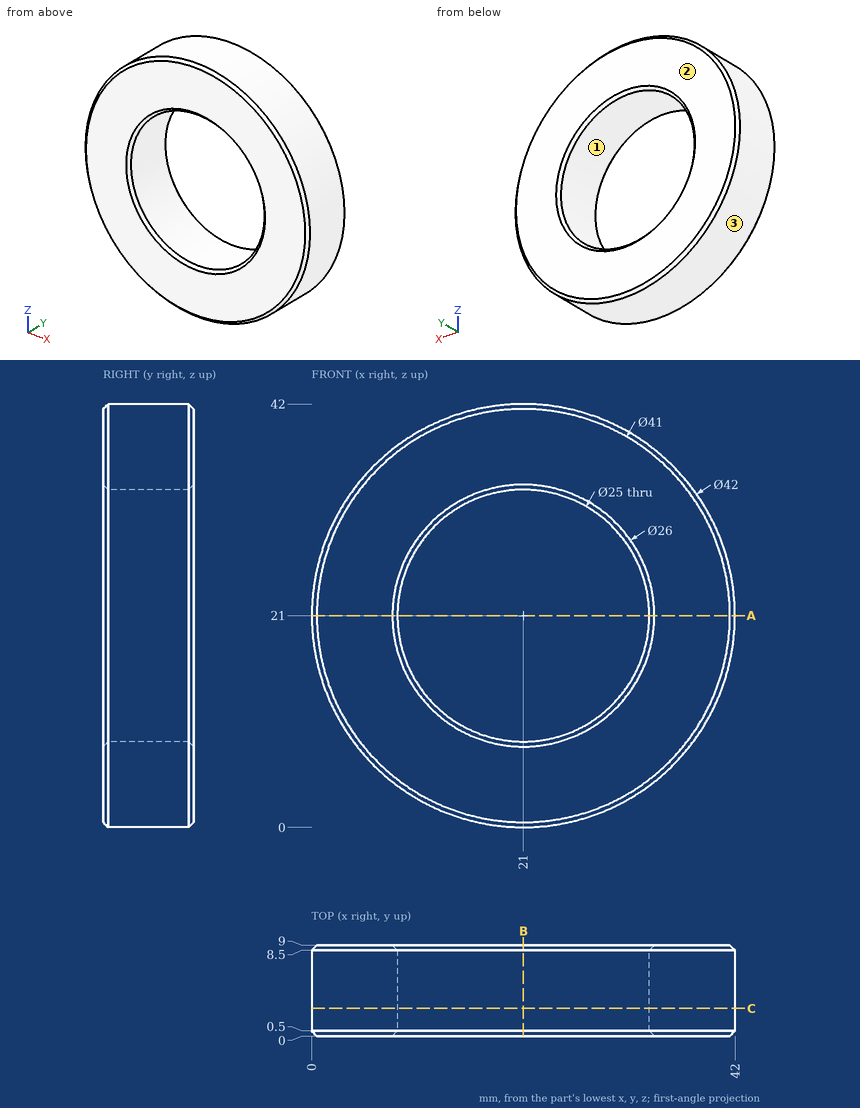
Study the drawing (mm; zero at the part's minimum x, y, z) and answer. Coordinates: 2 decimals unless noted, no trailing zeros. Order: outer loops, then holes, each group sorted by start corner. A loop starts at its lowest first (then second) coordinate and runs counter-clockwise, first axis right, second up. Notation, with made-up numbers: M 5.5,32.25 L 53.5,32.25 A20 ccw 53.5,54.25 Z; hole C -31.5,-25.5 d1. An arc over 180 degrees is marked long. Use CSV: the item, a comma, the result in double quotes.
Q1. Section B-B (x = 21) is taken. Determine the outline of the cut face in (y, z).
Here are the results:
outline,"M 0,0.5 L 0.5,0 L 8.5,0 L 9,0.5 L 9,8 L 8.5,8.5 L 0.5,8.5 L 0,8 Z; M 0,34 L 0.5,33.5 L 8.5,33.5 L 9,34 L 9,41.5 L 8.5,42 L 0.5,42 L 0,41.5 Z"
Q2. Straight lines are drawn through the part: L1, parallel to Z at x = 21, y = 3.75; L2, parallel to X at y = 2.5, z = 18; L3, parallel to Z at x = 15, y = 4.5. For each, find the intervals that lie inside material, in ascending order.
Here are the results:
L1,"0 to 8.5, 33.5 to 42"
L2,"0.22 to 8.87, 33.13 to 41.78"
L3,"0.88 to 10.03, 31.97 to 41.12"
Q3. Section C-C (y = 2.75) is taken. Determine the outline of the cut face in (x, z).
Here are the results:
outline,"C 21,21 d42; hole C 21,21 d25"
Q4. Given pin 1 Ø3 at (y, z) = (3.5, 7.5) entering from -X; pin 2 Ø1 at (x, y) = (15.5, 1) entering from -Z; pin 3 Ø2 at (x, y) = (31.5, 7) entering from +Z, each flat-ended and moving along its own axis, determine where each tip first touches the part or whether it passes through.
Here are the results:
pin 1,"x = 3.77"
pin 2,"z = 0.6"
pin 3,"z = 39.73"
Q5. Section A-A (z = 21) is taken. Determine the outline of the cut face in (x, y), then the cut area to 3 significant figures.
Here are the results:
outline,"M 0,0.5 L 0.5,0 L 8,0 L 8.5,0.5 L 8.5,8.5 L 8,9 L 0.5,9 L 0,8.5 Z; M 33.5,0.5 L 34,0 L 41.5,0 L 42,0.5 L 42,8.5 L 41.5,9 L 34,9 L 33.5,8.5 Z"
area,"152 mm2"
Q6. Determine the mould class of the marked faces 1, 2 and 3 for opening direction Z: pulls with the +Z half, pulls with the -Z half, needs draft (parallel to the pull), parting line crosses it, or undercut.
Here are the results:
face 1,"undercut"
face 2,"needs draft"
face 3,"parting line crosses it"
